Input: part model. Units: mm. Frame: model coordinates. A direction names the side the tool comes from. Coordinates: 2 decimals unless noted, no trailing zeros. Order: outer loops, then holes, each group sorted by start corner. A loop starts at its lowest first (then second) coordinate and runs counter-clockwise, first axis right, second up. Notation, with made-up numbers: (17.5, 51.25) - (52.5, 51.25) arc R11 cw to (52.5, 71.25) - close; hole circle Ø8 at (66, 15.5). An arc over 180 degrees is marked (long way). Use a Markdown table: item, result. Add a question column.
from build123d import *

# Parameters (mm, degrees)
SKETCH1_R           = 10
BOSS_EXTRUDE2_DEPTH = 10
CUT_EXTRUDE3_REACH  = 19.321
SKETCH5_R           = 1.5
SKETCH6_R           = 10
BOSS_EXTRUDE3_DEPTH = 5.75
SKETCH7_R           = 5
CUT_EXTRUDE4_DEPTH  = 5.75
SKETCH8_R           = 7.5
BOSS_EXTRUDE4_DEPTH = 10
SKETCH9_R           = 10
BOSS_EXTRUDE5_DEPTH = 5.75
CUT_EXTRUDE5_REACH  = 36.529
SKETCH10_R          = 5


with BuildPart() as part:
    # Sketch1 → Boss-Extrude2 (new body)
    with BuildSketch(Plane(origin=(0, 0, 0), x_dir=(1, 0, 0), z_dir=(0, 1, 0))):
        with Locations(Location((0, 0, 0), (0, 0, 270))):
            Circle(SKETCH1_R)
    extrude(amount=BOSS_EXTRUDE2_DEPTH)

    # Sketch5 → Cut-Extrude3 (cut, up to next)
    with BuildSketch(Plane(origin=(0, 10, 0), x_dir=(-1, 0, 0), z_dir=(0, 1, 0)), mode=Mode.PRIVATE) as cut_extrude3_sk1:
        with Locations(Location((0, 0, 0), (0, 0, 90))):
            Circle(SKETCH5_R)
    cut_extrude3_tool1 = extrude(cut_extrude3_sk1.sketch, amount=-CUT_EXTRUDE3_REACH, mode=Mode.PRIVATE) & part.part
    add(cut_extrude3_tool1.solids().sort_by_distance((0, 10, 0))[0], mode=Mode.SUBTRACT)

    # Sketch6 → Boss-Extrude3 (add)
    with BuildSketch(Plane(origin=(0, 10, 0), x_dir=(-1, 0, 0), z_dir=(0, 1, 0))):
        with Locations(Location((0, 0, 0), (0, 0, 90))):
            Circle(SKETCH6_R)
    extrude(amount=BOSS_EXTRUDE3_DEPTH)

    # Sketch7 → Cut-Extrude4 (cut)
    with BuildSketch(Plane(origin=(0, 15.75, 0), x_dir=(-1, 0, 0), z_dir=(0, 1, 0))):
        with Locations(Location((0, 0, 0), (0, 0, 90))):
            Circle(SKETCH7_R)
    extrude(amount=-CUT_EXTRUDE4_DEPTH, mode=Mode.SUBTRACT)

    # Sketch8 → Boss-Extrude4 (add)
    with BuildSketch(Plane(origin=(0, 15.75, 0), x_dir=(-1, 0, 0), z_dir=(0, 1, 0))):
        with Locations(Location((0, 0, 0), (0, 0, 90))):
            Circle(SKETCH8_R)
    extrude(amount=BOSS_EXTRUDE4_DEPTH)

    # Sketch9 → Boss-Extrude5 (add)
    with BuildSketch(Plane(origin=(0, 25.75, 0), x_dir=(-1, 0, 0), z_dir=(0, 1, 0))):
        with Locations(Location((0, 0, 0), (0, 0, 90))):
            Circle(SKETCH9_R)
    extrude(amount=BOSS_EXTRUDE5_DEPTH)

    # Sketch10 → Cut-Extrude5 (cut, up to next)
    with BuildSketch(Plane(origin=(0, 31.5, 0), x_dir=(-1, 0, 0), z_dir=(0, 1, 0)), mode=Mode.PRIVATE) as cut_extrude5_sk1:
        with Locations(Location((0, 0, 0), (0, 0, 90))):
            Circle(SKETCH10_R)
    cut_extrude5_tool1 = extrude(cut_extrude5_sk1.sketch, amount=-CUT_EXTRUDE5_REACH, mode=Mode.PRIVATE) & part.part
    add(cut_extrude5_tool1.solids().sort_by_distance((0, 31.5, 0))[0], mode=Mode.SUBTRACT)


solid = part.part
1) Cut plane C-C (y = 13). Return the cut outline in (x, z), and give its area (3 significant figures).
2) Contact query for flat-ended pins moving along their axis: P1, Ø5, axis at y = 17.5, z = 3, coming from the +X side; P2, Ø6, axis at y = 23, z = -6, coming from the +X side; P3, Ø5, axis at x = 7, y = 21, coming from the -Z side. Output: stop coordinate, or through.
3) Pull-direction query (Y, two-part tool) for faces 1 (the cylindrical face through (-4.88, 20.9, -1.08)), 2 (the flat face through (1.2, 10, -1.2)), 3 (the flat face through (7, 25.75, 4)); classes: pulls with the +Y half, pulls with the -Y half, needs draft (parallel to the pull), parting line crosses it, or undercut.
4) Cut plane A-A (z = 0). Return the cut outline in (x, y), and give its area (3 significant figures).
5) Reachability of faces 4 (the flat face through (5, 31.5, 2)), 5 (the cylindrical face through (0.33, 20.68, -7.493)) from +Z, -Z, +X, -X, +Y, -Y: full face, straight path, thin tool, end or side. Return the list, or none.
6) Cut plane B-B (x = 0). Return the cut outline in (y, z), and give its area (3 significant figures).
7) Cut plane D-D (z = -8). Return the cut outline in (x, y), and give its area (3 significant figures).
8) Material intervals for L1, parallel to X at y = 18.5, z = 0; L2, parallel to X at y = 5.75, z = 0; L3, parallel to Y at x = 8.75, z = 1.75, sorted ascending.
Computed:
| question | item | result |
|---|---|---|
| 1 | outline | circle Ø20 at (0, 0); hole circle Ø10 at (0, 0) |
| 1 | area | 236 mm2 |
| 2 | P1 | stops at x = 9.93 |
| 2 | P2 | stops at x = 8.77 |
| 2 | P3 | stops at z = -6 |
| 3 | face 1 | needs draft |
| 3 | face 2 | pulls with the +Y half |
| 3 | face 3 | undercut |
| 4 | outline | (-10, 0) - (-1.5, 0) - (-1.5, 10) - (-5, 10) - (-5, 31.5) - (-10, 31.5) - (-10, 25.75) - (-7.5, 25.75) - (-7.5, 15.75) - (-10, 15.75) - close; (1.5, 0) - (10, 0) - (10, 15.75) - (7.5, 15.75) - (7.5, 25.75) - (10, 25.75) - (10, 31.5) - (5, 31.5) - (5, 10) - (1.5, 10) - close |
| 4 | area | 335 mm2 |
| 5 | face 4 | +Z, -Z, +X, -X, +Y |
| 5 | face 5 | none |
| 6 | outline | (0, -10) - (15.75, -10) - (15.75, -7.5) - (25.75, -7.5) - (25.75, -10) - (31.5, -10) - (31.5, -5) - (10, -5) - (10, -1.5) - (0, -1.5) - close; (0, 1.5) - (10, 1.5) - (10, 5) - (31.5, 5) - (31.5, 10) - (25.75, 10) - (25.75, 7.5) - (15.75, 7.5) - (15.75, 10) - (0, 10) - close |
| 6 | area | 335 mm2 |
| 7 | outline | (-6, 0) - (6, 0) - (6, 15.75) - (-6, 15.75) - close; (-6, 25.75) - (6, 25.75) - (6, 31.5) - (-6, 31.5) - close |
| 7 | area | 258 mm2 |
| 8 | L1 | x = -7.5 to -5, 5 to 7.5 |
| 8 | L2 | x = -10 to -1.5, 1.5 to 10 |
| 8 | L3 | y = 0 to 15.75, 25.75 to 31.5 |
